Input: part model. Units: mm. Frame: model coordinates. Coordinates: 2 decimals unless noted, no trailing zeros. Loops run counter-clockwise (first coordinate to the right, second up) from the corner with the lowest first, then second, coordinate; pieces in that order, holes last.
Item 1: Section C-C on y = 0.2. Give the number of separate pieces and of enclosed holes in the cut face, and give its area (3 significant figures).
Item 2: Section B-B on x = 0. Return loops of the section in (y, z).
Item 3: Ray query, line 1 along Z through (x, y) = (0, 0.55); line 2 along Z through (x, y) = (-11.5, 0.15); line 3 along Z through (x, y) = (-1.5, 0.55). Return the intervals inside material, ascending.
Item 4: Pull-direction query (X, two-part tool) for faces 1 (the flat face through (8, 0, 8)), 2 (the cylindrical face through (-8.67, 0.49, 39.05)), 3 (the cylindrical face through (15.954, 0.507, -0.3)); classes: released by +X, released by -X, zero draft, split by the parting line, or undercut.
Item 5: Section A-A on z = 0. Return loops of the section in (x, y).
Item 6: Section D-D on x = 8. Return loops of the section in (y, z).
```python
from build123d import *

# Parameters (mm, degrees)
SKETCH2_R           = 40
BOSS_EXTRUDE1_DEPTH = 1
SKETCH3_R           = 10
CUT_EXTRUDE1_DEPTH  = 2
SKETCH4_R           = 1
CUT_EXTRUDE2_DEPTH  = 2


with BuildPart() as part:
    # Sketch2 → Boss-Extrude1 (new body)
    with BuildSketch(Plane(origin=(0, 0, 0), x_dir=(1, 0, 0), z_dir=(0, 1, 0))):
        Circle(SKETCH2_R)
    extrude(amount=BOSS_EXTRUDE1_DEPTH)

    # Sketch3 → Cut-Extrude1 (cut, through all)
    with BuildSketch(Plane(origin=(0, 1, 0), x_dir=(1, 0, 0), z_dir=(0, 1, 0))):
        Circle(SKETCH3_R)
    extrude(amount=-CUT_EXTRUDE1_DEPTH, mode=Mode.SUBTRACT)

    # Sketch4 → Cut-Extrude2 (cut, through all)
    with BuildSketch(Plane(origin=(0, 1, 0), x_dir=(1, 0, 0), z_dir=(0, 1, 0))):
        with Locations((0, 15)):
            Circle(SKETCH4_R)
        with Locations((10.606601718, 10.606601718)):
            Circle(SKETCH4_R)
        with Locations((15, 0)):
            Circle(SKETCH4_R)
        with Locations((10.606601718, -10.606601718)):
            Circle(SKETCH4_R)
        with Locations((0, -15)):
            Circle(SKETCH4_R)
        with Locations((-10.606601718, -10.606601718)):
            Circle(SKETCH4_R)
        with Locations((-15, 0)):
            Circle(SKETCH4_R)
        with Locations((-10.606601718, 10.606601718)):
            Circle(SKETCH4_R)
    extrude(amount=-CUT_EXTRUDE2_DEPTH, mode=Mode.SUBTRACT)


solid = part.part
```
Results found:
1. separate pieces: 1
1. enclosed holes: 9
1. area: 4,690 mm2
2. outline: (0, -40) - (1, -40) - (1, -16) - (0, -16) - close; (0, -14) - (1, -14) - (1, -10) - (0, -10) - close; (0, 10) - (1, 10) - (1, 14) - (0, 14) - close; (0, 16) - (1, 16) - (1, 40) - (0, 40) - close
3. line 1: z = -40 to -16, -14 to -10, 10 to 14, 16 to 40
3. line 2: z = -38.31 to -11.06, -10.16 to 10.16, 11.06 to 38.31
3. line 3: z = -39.97 to -9.89, 9.89 to 39.97
4. face 1: zero draft
4. face 2: split by the parting line
4. face 3: undercut
5. outline: (-40, 0) - (-16, 0) - (-16, 1) - (-40, 1) - close; (-14, 0) - (-10, 0) - (-10, 1) - (-14, 1) - close; (10, 0) - (14, 0) - (14, 1) - (10, 1) - close; (16, 0) - (40, 0) - (40, 1) - (16, 1) - close
6. outline: (0, -39.19) - (1, -39.19) - (1, -6) - (0, -6) - close; (0, 6) - (1, 6) - (1, 39.19) - (0, 39.19) - close
